from build123d import *

# Parameters (mm, degrees)
EXTRUDE_2_DEPTH     = 40
SKETCH_3_R          = 1.5
CUT_EXTRUDE_1_DEPTH = 10
SKETCH_4_R          = 1.686195938
SKETCH_4_R_2        = 1.862668349
CUT_EXTRUDE_2_DEPTH = 10


with BuildPart() as part:
    # 草图2 → 凸台-拉伸2 (new body)
    with BuildSketch(Plane.XY):
        Polygon((0, 0), (0, 10), (8, 18), (11, 18), (3, 10), (3, 0), align=None)
    extrude(amount=EXTRUDE_2_DEPTH)

    # 草图3 → 切除-拉伸1 (cut)
    with BuildSketch(Plane(origin=(3, 0, 0), x_dir=(0, 0, -1), z_dir=(1, 0, 0))):
        with Locations(Location((-10, 5, 0), (0, 0, 90))):
            Circle(SKETCH_3_R)
        with Locations(Location((-30, 5, 0), (0, 0, 90))):
            Circle(SKETCH_3_R)
    extrude(amount=-CUT_EXTRUDE_1_DEPTH, mode=Mode.SUBTRACT)

    # 草图4 → 切除-拉伸2 (cut)
    with BuildSketch(Plane(origin=(-3.5, 3.5, 0), x_dir=(0, 0, -1), z_dir=(0.7071067811865515, -0.7071067811865437, 0))):
        with Locations(Location((-7, 15.192388155, 0), (0, 0, 90))):
            Circle(SKETCH_4_R)
        with Locations(Location((-33, 15.192388155, 0), (0, 0, 90))):
            Circle(SKETCH_4_R_2)
    extrude(amount=-CUT_EXTRUDE_2_DEPTH, mode=Mode.SUBTRACT)


solid = part.part
Build history of the part. All positions in model axes, mm. A direction names the side the tool comes from. Coordinates: 2 decimals unless noted, no trailing zeros. Write each loop counter-clockwise with the first axis right and the second up, starting at its lowest first coordinate (ties: lowest second). Pieces come first, ordered by that corner, then holes.
(1) Drill centre lines: line 1 (Z direction, x = 2.1, y = 5); line 2 (Z direction, x = 0.75, y = 4.5); line 3 (X direction, y = 4.5, z = 6.5). Where is each one in solid material? Low to high.
(2) Cut at B-B on z = 10. List the corners of the cut face in (x, y), and give its area (3 significant figures).
(3) Pin check, flat tips, straight feed: pin 1 Ø3 at (y, z) = (4, 10) entering from +X; pin 2 Ø5 at (x, y) = (6.5, 7) entering from -Z; pin 3 Ø2 at (y, z) = (11, 34) entering from +X; pin 4 Ø8 at (y, z) = (6.5, 7) entering from +X. Stop position of each tip, or through.
(4) 3-axis set-ups, long thin cutter, end or side, ignore diameter. For faces 1 (the flat face through (3, 5, 20)), 2 (the flat face through (9, 18, 20)): which of +Z, -Z, +X, -X, +Y, -Y reach the whole face in a straight line?
(5) Cut at D-D on z = 38.5. List the corners of the cut face in (x, y), and give its area (3 significant figures).
(6) Cut at A-A on y = 5. List the corners of the cut face in (x, z), and give its area (3 significant figures).
(7) Mould opens along Z. For faces 3 (the cylindrical face through (7.144, 15.623, 8.422)), 4 (the flat face through (2, 0, 20)), 5 (the flat face through (2.7, 9, 40)) say: pulls with the +Z half, pulls with the -Z half, needs draft (parallel to the pull), parting line crosses it, or undercut.
(8) Cut at C-C on x = 2.5. List the corners of the cut face in (y, z), and give its area (3 significant figures).
Working result:
1. line 1: z = 0 to 8.5, 11.5 to 28.5, 31.5 to 40
1. line 2: z = 0 to 8.59, 11.41 to 28.59, 31.41 to 40
1. line 3: x = 0 to 3
2. outline: (0, 0) - (3, 0) - (3, 3.5) - (0, 3.5) - close; (0, 6.5) - (3, 6.5) - (3, 10) - (11, 18) - (8, 18) - (0, 10) - close
2. area: 45.0 mm2
3. pin 1: stops at x = 3
3. pin 2: passes through
3. pin 3: stops at x = 5
3. pin 4: stops at x = 3.5
4. face 1: +Z, -Z, +X, -Y
4. face 2: +Z, -Z, +X, -X, +Y
5. outline: (0, 0) - (3, 0) - (3, 10) - (11, 18) - (8, 18) - (0, 10) - close
5. area: 54.0 mm2
6. outline: (0, 0) - (3, 0) - (3, 8.5) - (0, 8.5) - close; (0, 11.5) - (3, 11.5) - (3, 28.5) - (0, 28.5) - close; (0, 31.5) - (3, 31.5) - (3, 40) - (0, 40) - close
6. area: 102 mm2
7. face 3: undercut
7. face 4: needs draft
7. face 5: pulls with the +Z half
8. outline: (0, 0) - (12.5, 0) - (12.5, 40) - (0, 40) - close; hole circle Ø3 at (5, 10); hole circle Ø3 at (5, 30)
8. area: 486 mm2
